```python
from build123d import *

# Parameters (mm, degrees)
SKETCH1_W             = 16
SKETCH1_H             = 28.5
BOSS_EXTRUDE1_DEPTH   = 3
CAVITY1_START         = 23.498167492
CAVITY1_OUTLINE_W     = 10.447458445
CAVITY1_OUTLINE_H     = 3
CAVITY1_OUTLINE_W_2   = 8.052541555
CAVITY1_DEPTH         = 3
CAVITY1_START_2       = 36.498167492
CAVITY1_2_OUTLINE_W   = 10.447458445
CAVITY1_2_OUTLINE_H   = 3
CAVITY1_2_OUTLINE_W_2 = 8.052541555
CAVITY1_2_DEPTH       = 3
CAVITY1_START_3       = 26.498167492
CAVITY1_3_OUTLINE_W   = 3
CAVITY1_3_OUTLINE_H   = 3
CAVITY1_3_DEPTH       = 2.5
CAVITY1_START_4       = 33.998167492
CAVITY1_4_OUTLINE_W   = 3
CAVITY1_4_OUTLINE_H   = 3
CAVITY1_4_DEPTH       = 2.5


# Read off the part's stored shape, not the designer's step: Cavity1
with BuildPart() as part:
    # Sketch1 → Boss-Extrude1 (new body)
    with BuildSketch(Plane.XY):
        with Locations((31.498167492, 24.589698152)):
            Rectangle(SKETCH1_W, SKETCH1_H)
    extrude(amount=BOSS_EXTRUDE1_DEPTH)

    # Cavity1 outline → Cavity1 (cut)
    with BuildSketch(Plane.YZ.offset(CAVITY1_START)):
        with Locations((33.615968929, 1.5)):
            Rectangle(CAVITY1_OUTLINE_W, CAVITY1_OUTLINE_H)
        with Locations((14.36596893, 1.5)):
            Rectangle(CAVITY1_OUTLINE_W_2, CAVITY1_OUTLINE_H)
    extrude(amount=CAVITY1_DEPTH, mode=Mode.SUBTRACT)

    # Cavity1 2 outline → Cavity1 2 (cut)
    with BuildSketch(Plane.YZ.offset(CAVITY1_START_2)):
        with Locations((33.615968929, 1.5)):
            Rectangle(CAVITY1_2_OUTLINE_W, CAVITY1_2_OUTLINE_H)
        with Locations((14.36596893, 1.5)):
            Rectangle(CAVITY1_2_OUTLINE_W_2, CAVITY1_2_OUTLINE_H)
    extrude(amount=CAVITY1_2_DEPTH, mode=Mode.SUBTRACT)

    # Cavity1 3 outline → Cavity1 3 (cut)
    with BuildSketch(Plane.YZ.offset(CAVITY1_START_3)):
        with Locations((37.339698152, 1.5)):
            Rectangle(CAVITY1_3_OUTLINE_W, CAVITY1_3_OUTLINE_H)
    extrude(amount=CAVITY1_3_DEPTH, mode=Mode.SUBTRACT)

    # Cavity1 4 outline → Cavity1 4 (cut)
    with BuildSketch(Plane.YZ.offset(CAVITY1_START_4)):
        with Locations((37.339698152, 1.5)):
            Rectangle(CAVITY1_4_OUTLINE_W, CAVITY1_4_OUTLINE_H)
    extrude(amount=CAVITY1_4_DEPTH, mode=Mode.SUBTRACT)


solid = part.part
```
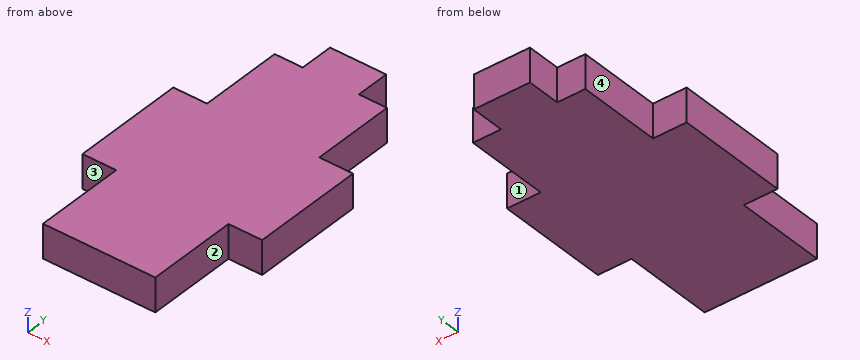
For this review, take the finished solid that the model builds, in its own axes (mm). Face numbers are marked on the shaded views. A direction names the side the tool comes from. Round coordinates to 2 decimals unless told otherwise and drop trailing zeros. Write each loop counter-clockwise with the first axis right and the second up, starting at its lowest first coordinate (ties: lowest second). Pieces come first, ordered by that corner, then holes. Notation, with made-up numbers: (70.5, 63.5) -> (96.5, 63.5) arc R32 cw to (96.5, 97.5) -> close; hole circle Ø9 at (16, 42). An arc over 180 degrees is marked (long way). Use one line per item in the form item = value.
Q1. Machinability: for the marked faces 1, 2, 3 and 4, which of the approach directions +Z, -Z, +X, -X, +Y, -Y give a long, thin tool a straight path to every point of the face, cutting with its end or side? Answer none if there is none.
Resolved:
face_1 = +Z, -Z, +X, +Y
face_2 = +Z, -Z, +X, -Y
face_3 = +Z, -Z, -X, -Y
face_4 = +Z, -Z, -X, +Y
Q2. Consider section A-A (z = 1.1). State the section outline as (x, y) points.
Resolved:
outline = (23.5, 18.39) -> (26.5, 18.39) -> (26.5, 10.34) -> (36.5, 10.34) -> (36.5, 18.39) -> (39.5, 18.39) -> (39.5, 28.39) -> (36.5, 28.39) -> (36.5, 35.84) -> (34, 35.84) -> (34, 38.84) -> (29, 38.84) -> (29, 35.84) -> (26.5, 35.84) -> (26.5, 28.39) -> (23.5, 28.39) -> close
Q3. To check wall thickness, follow probe 1 along X at (y, z) = (28.5, 1.6); probe 2 along Y at (x, z) = (24.5, 0.55); probe 3 along Y at (x, z) = (28.25, 0.95). State the ranges of each line that lie inside material, in increasing order. Write a range as from..to.
Resolved:
probe_1 = 26.5..36.5
probe_2 = 18.39..28.39
probe_3 = 10.34..35.84
Q4. Clearance check with flat-ended pins moving along their axes: pin 1 Ø0.9 at (x, z) = (25.5, 2) entering from +Y; pin 2 Ø1.5 at (y, z) = (33, 1.5) entering from -X; pin 3 Ø1.5 at (y, z) = (37.5, 2) entering from -X; pin 4 Ø1 at (x, y) = (38, 29.5) entering from +Z. State where each tip first meets the part, or that it passes through.
Resolved:
pin_1 = 28.39
pin_2 = 26.5
pin_3 = 29
pin_4 = through
Q5. Consider section C-C (x = 27). State the section outline as (y, z) points.
Resolved:
outline = (10.34, 0) -> (35.84, 0) -> (35.84, 3) -> (10.34, 3) -> close
Q6. Consider section B-B (y = 15.75). State the section outline as (x, z) points, then the cut area to 3 significant figures.
Resolved:
outline = (26.5, 0) -> (36.5, 0) -> (36.5, 3) -> (26.5, 3) -> close
area = 30.0 mm²
